Can you work these out from the model? Positions are in its coordinate system, mm. A direction names the side the tool comes from. Give positions to 0.01 mm unless a question says otherwise; leave off trailing zeros. Loops run counter-clockwise (first coordinate to the right, second up) from the corner with the lowest first, then second, coordinate; pieces in that order, holes last. Notation, with made-up numbers: (12.25, 61.5) -> (49.25, 61.5) arc R21 cw to (49.25, 68.5) -> close; hole circle Ø8 at (81.5, 24). An arc over 180 degrees is marked (long way). Return JSON: item names as keys, results as strings. Group by question number.
Q1. Suppose I cut it at D-D, the plane x = 2. Please give me the cut outline in (y, z).
Q2. Will these pins go through, and if not, where does the flat tip stop? pin 1 (0.8 mm diameter, centred on x = 0, y = -6, fed in from +Z); pin 2 (1.6 mm diameter, centred on x = 2, y = -5.5, fed in from -Z); pin 3 (0.5 mm diameter, centred on x = -1.5, z = 6.5, fed in from -Y).
Q3. Suppose I cut it at A-A, the plane x = -1. Please give me the cut outline in (y, z), and give its area (3 significant figures).
Q4. Suppose I cut it at B-B, the plane y = -0.75. Please give me the cut outline in (x, z), and give its area (3 significant figures).
Q5. I need wall thicknesses on line 1 along X through (y, z) = (-3.25, 4.5); line 2 along Y through (x, z) = (-1.5, -6.25); line 3 along Z through (x, y) = (1, -4.5). Which ranges of each line are inside material? Lowest first, please. Write a range as [from, to].
Q6. Suppose I cut it at C-C, the plane z = 5.5. Please give me the cut outline in (x, y), and give its area (3 significant figures).
Q7. Which directions (+Z, -Z, +X, -X, +Y, -Y) give clear straight access to the entire face, cutting with the end or side of a thin tool? Please do faces 5 (the flat face through (0.1, -0.41, -6.5)), 6 (the flat face through (3.75, -5.2, 0.4)), 7 (the flat face through (0, -6, -6.204)).
Q8. Thinking about a two-plate mould opening in Y: for faces 1 (the flat face through (0, -6.5, 0)), 2 (the flat face through (-1, 0, 6)), 3 (the flat face through (0, -5, 5)), 4 (the flat face through (-3.75, -3, 0)), which applies, pulls with the +Y half, pulls with the -Y half, needs draft (parallel to the pull), parting line crosses it, or undercut?
```python
from build123d import *

# Parameters (mm, degrees)
BOSS_EXTRUDE1_DEPTH = 4
CUT_EXTRUDE1_DEPTH  = 3.75
CUT_EXTRUDE2_REACH  = 14.46
CUT_EXTRUDE3_REACH  = 14.301
CUT_EXTRUDE4_REACH  = 12.356
SKETCH6_R           = 0.205


with BuildPart() as part:
    # Sketch1 → Boss-Extrude1 (new, symmetric)
    with BuildSketch(Plane(origin=(0, 0, 0), x_dir=(0, 0, -1), z_dir=(1, 0, 0))):
        with BuildLine():
            Line((-7, 0), (7, 0))
            Line((7, 0), (7, -0.41))
            Line((7, -0.41), (5.985975276, -0.41))
            ThreePointArc((5.985975276, -0.41), (5.186676874, -3.016352599), (3.31662479, -5))
            Line((3.31662479, -5), (6.203592814, -5))
            Line((6.203592814, -5), (6.203592814, -6.5))
            Line((6.203592814, -6.5), (-5.910179641, -6.5))
            Line((-5.910179641, -6.5), (-5.910179641, -5))
            Line((-5.910179641, -5), (-3.31662479, -5))
            ThreePointArc((-3.31662479, -5), (-5.186676874, -3.016352599), (-5.985975276, -0.41))
            Line((-5.985975276, -0.41), (-7, -0.41))
            Line((-7, -0.41), (-7, 0))
        make_face()
    extrude(amount=BOSS_EXTRUDE1_DEPTH, both=True)

    # Sketch2 → Cut-Extrude1 (cut, symmetric)
    with BuildSketch(Plane(origin=(0, 0, 0), x_dir=(0, 0, -1), z_dir=(1, 0, 0))):
        with BuildLine():
            Line((-5.75, 0), (5.75, 0))
            ThreePointArc((5.75, 0), (0, -5.75), (-5.75, 0))
        make_face()
    extrude(amount=CUT_EXTRUDE1_DEPTH, both=True, mode=Mode.SUBTRACT)

    # Sketch3 → Cut-Extrude2 (cut, up to next)
    with BuildSketch(Plane(origin=(4, 0, 0), x_dir=(0, 0, -1), z_dir=(1, 0, 0)), mode=Mode.PRIVATE) as cut_extrude2_sk1:
        with BuildLine():
            Line((-4.875, 0), (4.875, 0))
            ThreePointArc((4.875, 0), (0, -4.875), (-4.875, 0))
        make_face()
    cut_extrude2_tool1 = extrude(cut_extrude2_sk1.sketch, amount=-CUT_EXTRUDE2_REACH, mode=Mode.PRIVATE) & part.part
    add(cut_extrude2_tool1.solids().sort_by_distance((4, -2.069014, 0))[0], mode=Mode.SUBTRACT)

    # Sketch4 → Cut-Extrude3 (cut, up to next)
    with BuildSketch(Plane(origin=(-3.75, 0, 0), x_dir=(0, 0, -1), z_dir=(1, 0, 0)), mode=Mode.PRIVATE) as cut_extrude3_sk1:
        with BuildLine():
            Line((-1.5, 0), (1.5, 0))
            ThreePointArc((1.5, 0), (0, -1.5), (-1.5, 0))
        make_face()
    cut_extrude3_tool1 = extrude(cut_extrude3_sk1.sketch, amount=-CUT_EXTRUDE3_REACH, mode=Mode.PRIVATE) & part.part
    add(cut_extrude3_tool1.solids().sort_by_distance((-3.75, -0.63662, 0))[0], mode=Mode.SUBTRACT)

    # Sketch6 → Cut-Extrude4 (cut, up to next)
    with BuildSketch(Plane(origin=(0, 0, 0), x_dir=(1, 0, 0), z_dir=(0, 1, 0)), mode=Mode.PRIVATE) as cut_extrude4_sk1:
        with Locations(Location((3, 6.357400892, 0), (0, 0, 270))):
            Circle(SKETCH6_R)
    cut_extrude4_tool1 = extrude(cut_extrude4_sk1.sketch, amount=-CUT_EXTRUDE4_REACH, mode=Mode.PRIVATE) & part.part
    # Sketch6 → Cut-Extrude4 (cut, up to next)
    with BuildSketch(Plane(origin=(0, 0, 0), x_dir=(1, 0, 0), z_dir=(0, 1, 0)), mode=Mode.PRIVATE) as cut_extrude4_sk2:
        with Locations(Location((1, 6.357400892, 0), (0, 0, 270))):
            Circle(SKETCH6_R)
    cut_extrude4_tool2 = extrude(cut_extrude4_sk2.sketch, amount=-CUT_EXTRUDE4_REACH, mode=Mode.PRIVATE) & part.part
    # Sketch6 → Cut-Extrude4 (cut, up to next)
    with BuildSketch(Plane(origin=(0, 0, 0), x_dir=(1, 0, 0), z_dir=(0, 1, 0)), mode=Mode.PRIVATE) as cut_extrude4_sk3:
        with Locations(Location((-1, 6.357400892, 0), (0, 0, 270))):
            Circle(SKETCH6_R)
    cut_extrude4_tool3 = extrude(cut_extrude4_sk3.sketch, amount=-CUT_EXTRUDE4_REACH, mode=Mode.PRIVATE) & part.part
    # Sketch6 → Cut-Extrude4 (cut, up to next)
    with BuildSketch(Plane(origin=(0, 0, 0), x_dir=(1, 0, 0), z_dir=(0, 1, 0)), mode=Mode.PRIVATE) as cut_extrude4_sk4:
        with Locations(Location((-3, 6.357400892, 0), (0, 0, 270))):
            Circle(SKETCH6_R)
    cut_extrude4_tool4 = extrude(cut_extrude4_sk4.sketch, amount=-CUT_EXTRUDE4_REACH, mode=Mode.PRIVATE) & part.part
    cut_extrude4_1 = cut_extrude4_tool1.solids().sort_by_distance((3, 0, -6.357401))[0]
    add(cut_extrude4_1, mode=Mode.SUBTRACT)
    cut_extrude4_2 = cut_extrude4_tool2.solids().sort_by_distance((1, 0, -6.357401))[0]
    add(cut_extrude4_2, mode=Mode.SUBTRACT)
    cut_extrude4_3 = cut_extrude4_tool3.solids().sort_by_distance((-1, 0, -6.357401))[0]
    add(cut_extrude4_3, mode=Mode.SUBTRACT)
    cut_extrude4_4 = cut_extrude4_tool4.solids().sort_by_distance((-3, 0, -6.357401))[0]
    add(cut_extrude4_4, mode=Mode.SUBTRACT)
    cut_extrude4 = cut_extrude4_1 + cut_extrude4_2 + cut_extrude4_3 + cut_extrude4_4  # Cut-Extrude4 as one shape, for the pattern or mirror that repeats it

    # Mirror1: Cut-Extrude4 across plane
    add(cut_extrude4.mirror(Plane.XY), mode=Mode.SUBTRACT)


solid = part.part
```
Ans:
{
 "1": {"outline": "(-6.5, -6.2) -> (-5, -6.2) -> (-5, -3.32) arc R6 ccw to (-0.41, -5.99) -> (-0.41, -7) -> (0, -7) -> (0, -5.75) arc R5.75 cw to (0, 5.75) -> (0, 7) -> (-0.41, 7) -> (-0.41, 5.99) arc R6 ccw to (-5, 3.32) -> (-5, 5.91) -> (-6.5, 5.91) -> close"},
 "2": {"pin 1": "stops at z = 5.91", "pin 2": "stops at z = -6.2", "pin 3": "stops at y = -0.41"},
 "3": {"outline": "(-6.5, -6.2) -> (-5, -6.2) -> (-5, -3.32) arc R6 ccw to (-0.41, -5.99) -> (-0.41, -6.15) -> (0, -6.15) -> (0, -5.75) arc R5.75 cw to (0, 5.75) -> (0, 6.15) -> (-0.41, 6.15) -> (-0.41, 5.99) arc R6 ccw to (-5, 3.32) -> (-5, 5.91) -> (-6.5, 5.91) -> close; (-0.41, -7) -> (0, -7) -> (0, -6.56) -> (-0.41, -6.56) -> close; (-0.41, 6.56) -> (0, 6.56) -> (0, 7) -> (-0.41, 7) -> close", "area": "18.8 mm^2"},
 "4": {"outline": "(-4, -5.95) -> (4, -5.95) -> (4, -4.82) -> (3.75, -4.82) -> (3.75, -5.7) -> (-3.75, -5.7) -> (-3.75, -1.3) -> (-4, -1.3) -> close; (-4, 1.3) -> (-3.75, 1.3) -> (-3.75, 5.7) -> (3.75, 5.7) -> (3.75, 4.82) -> (4, 4.82) -> (4, 5.95) -> (-4, 5.95) -> close", "area": "6.68 mm^2"},
 "5": {"line 1": "x = [-4, -3.75], [3.75, 4]", "line 2": "y = [-0.41, 0]", "line 3": "z = [-3.97, -3.58], [3.58, 3.97]"},
 "6": {"outline": "(-4, -6.5) -> (4, -6.5) -> (4, -5) -> (-4, -5) -> close; (-4, -2.4) -> (4, -2.4) -> (4, 0) -> (3.75, 0) -> (3.75, -1.68) -> (-3.75, -1.68) -> (-3.75, 0) -> (-4, 0) -> close", "area": "18.6 mm^2"},
 "7": {"face 5": "-Z, +X, -X", "face 6": "+Y", "face 7": "-Z, +X, -X, -Y"},
 "8": {"face 1": "pulls with the -Y half", "face 2": "pulls with the +Y half", "face 3": "undercut", "face 4": "needs draft"}
}
